Answer from the drawing. Dimensions are ordinates in mm from the lowest x, y and z of the part. A direction names the side the tool comes from. Coordinates: 2 decimals unless noted, no trailing zeros. Write each loop counter-clockwise with the first axis right and the second up, starting at its lowest first coordinate (ties: lowest second). Pieces come first, ordered by that corner, then holes.
(1) Straight lines are drawn through the part: line 1 (X direction, y = 15, z = 0.3); line 2 (Y direction, x = 16.5, z = 2.1) (1 decimal); line 3 (X direction, y = 17.75, z = 1.95). For each, find the intervals that lie inside material, in ascending order.
(2) Given P1, Ø2, axis at x = 5, z = 1.5, coming from the -Y side; P2, Ø2, axis at y = 17, z = 1.5, coming from the -X side, each flat-ended and moving along its own axis, determine where each tip first touches the part or whether it passes through.
(3) The part is cut by section A-A on x = 15.5. Determine the outline of the cut face in (y, z).
(4) The part is cut by section C-C on y = 5.5. Determine the outline of the cut face in (x, z).
(5) The part is cut by section D-D on x = 5.5. Determine the outline of the cut face in (y, z) (1 decimal).
(6) For a pull along Y with two mould halves and no side action, classify the marked faces 1, 2 and 3 as +Y half, -Y half, draft (parallel to the pull), parting line (faces both ways), or undercut.
(7) The part is cut by section B-B on z = 3.3. Determine the outline of the cut face in (x, y).
(8) Which of the six approach directions +Z, -Z, +X, -X, +Y, -Y give full straight-line access (tool end or side, diameter ignored) to the marked faces 4, 5 and 6?
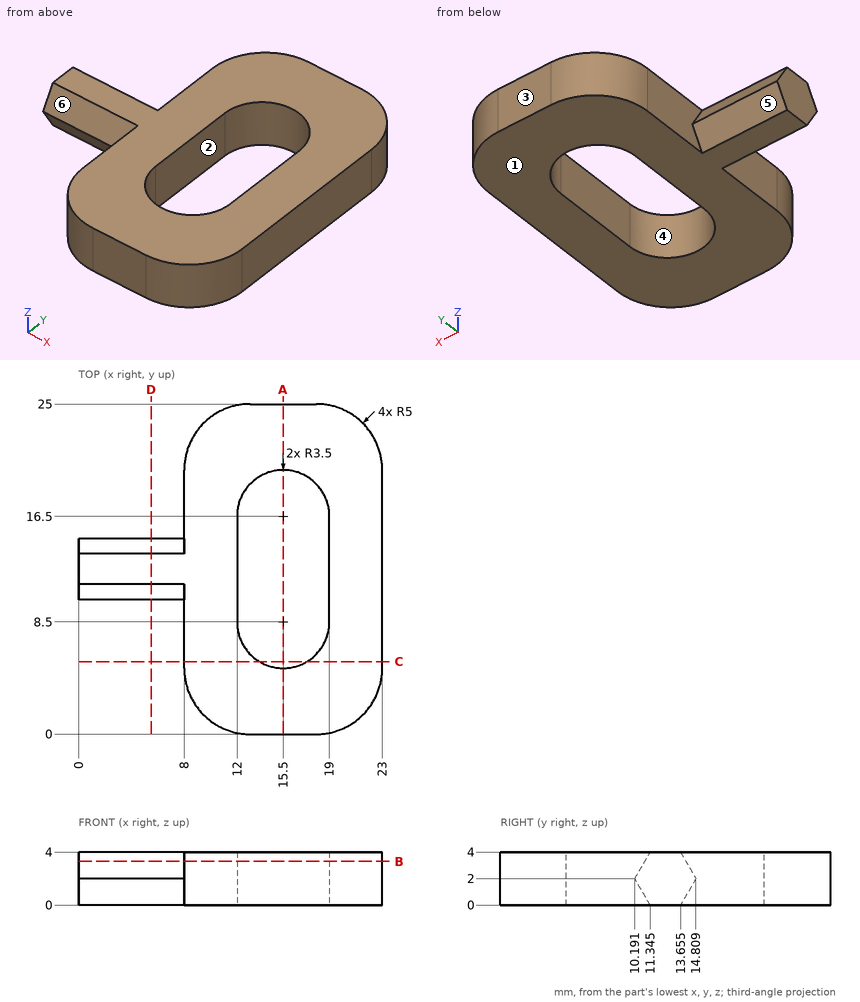
Model answer:
1. line 1: x = 8 to 12, 19 to 23
1. line 2: y = 0 to 5.1, 19.9 to 25
1. line 3: x = 8 to 12.23, 18.77 to 23
2. P1: stops at y = 10.19
2. P2: stops at x = 8
3. outline: (0, 0) - (5, 0) - (5, 4) - (0, 4) - close; (20, 0) - (25, 0) - (25, 4) - (20, 4) - close
4. outline: (8, 0) - (13.7, 0) - (13.7, 4) - (8, 4) - close; (17.3, 0) - (23, 0) - (23, 4) - (17.3, 4) - close
5. outline: (10.2, 2) - (11.3, 0) - (13.7, 0) - (14.8, 2) - (13.7, 4) - (11.3, 4) - close
6. face 1: draft
6. face 2: undercut
6. face 3: +Y half
7. outline: (0, 10.94) - (8, 10.94) - (8, 5) arc R5 ccw to (13, 0) - (18, 0) arc R5 ccw to (23, 5) - (23, 20) arc R5 ccw to (18, 25) - (13, 25) arc R5 ccw to (8, 20) - (8, 14.06) - (0, 14.06) - close; hole (12, 8.5) arc R3.5 ccw to (19, 8.5) - (19, 16.5) arc R3.5 ccw to (12, 16.5) - close
8. face 4: +Z, -Z
8. face 5: -Z, -X, +Y
8. face 6: +Z, -X, -Y
